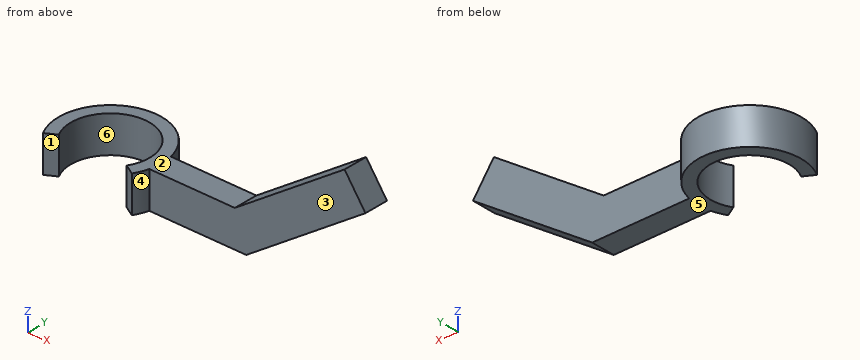
```python
from build123d import *

# Parameters (mm, degrees)
F2_DEPTH  = 15
F11_W     = 60
F11_H     = 10
F12_DEPTH = 15


with BuildPart() as f2:
    # F1 (on Top) → F2 (new body)
    with BuildSketch(Plane.XY):
        with BuildLine():
            ThreePointArc((-13.9863102711, -8.075), (0, 16.15), (13.9863102711, -8.075))
            Line((13.9863102711, -8.075), (18.31643729, -10.575))
            ThreePointArc((18.31643729, -10.575), (19.6323610311, -7.8672040995), (20.5504866122, -5))
            ThreePointArc((20.5504866122, -5), (21.15, 0), (20.5504866122, 5))
            ThreePointArc((20.5504866122, 5), (-7.8672040995, 19.6323610311), (-18.31643729, -10.575))
            Line((-18.31643729, -10.575), (-13.9863102711, -8.075))
        make_face()
        with BuildLine():
            ThreePointArc((20.5504866122, 5), (21.15, 0), (20.5504866122, -5))
            Line((20.5504866122, -5), (60.5504866122, -5))
            Line((60.5504866122, -5), (60.5504866122, 5))
            Line((60.5504866122, 5), (20.5504866122, 5))
        make_face()
    extrude(amount=F2_DEPTH)

    # F11 (on 3pt) → F12 (join)
    with BuildSketch(Plane(origin=(19.9205002513, 0, -28.4494227273), x_dir=(0.8191520443, 0, 0.5735764364), z_dir=(-0.5735764364, 0, 0.8191520443))):
        with Locations((79.6000548911, 0)):
            Rectangle(F11_W, F11_H)
    extrude(amount=F12_DEPTH)


solid = f2.part
```
Can you work these out from the model? Positions are in its coordinate system, mm. Face numbers are marked on the shaded views. A direction names the side the tool comes from. Coordinates: 2 decimals unless noted, no trailing zeros. Loops run counter-clockwise (first coordinate to the right, second up) from the corner with the lowest first, then second, coordinate; pieces in that order, holes last. Notation, with made-up numbers: (-28, 67.5) -> (30, 67.5) arc R5 cw to (30, 72.5) -> close; hole circle Ø11 at (32.25, -21.5). An arc over 180 degrees is marked (long way). Answer as a JSON object with one key per item and string values.
1) Imagine slicing it at C-C (z = 9). Please give me the cut outline in (x, y) (3 decimals).
Results:
{"outline": "(-18.316, -10.575) -> (-13.986, -8.075) arc R16.15 cw (long way) to (13.986, -8.075) -> (18.316, -10.575) arc R21.15 ccw to (20.55, -5) -> (73.404, -5) -> (73.404, 5) -> (20.55, 5) arc R21.15 ccw (long way) to start"}
2) For the marked faces 1, 2 and 3, which set-ups out of +Z, -Z, +X, -X, +Y, -Y let a thin tool reach every point of the face, with its end or its side?
Results:
{"face 1": "+Z, -Z, -Y", "face 2": "+Z, -X, +Y, -Y", "face 3": "+Z, -Z, +X, -Y"}
3) For P1, Ø14, axis at x = 54.5, z = 22, coming from the -Y side; P2, Ø12, axis at y = 15.5, z = 14, coming from the +X side; P3, Ø1, axis at y = 5, z = 16.5, coming from the +X side; P4, Ø6, axis at x = -5.5, y = 16.5, coming from the -Z side, each with a flat end and sliding along its axis, tell me the tip position at first contact or that it passes through.
Results:
{"P1": "stops at y = -5", "P2": "stops at x = 18.9", "P3": "stops at x = 84.83", "P4": "stops at z = 0"}
4) Imagine slicing it at D-D (y = 14). Please give me the cut outline in (x, z), then the cut area to 3 significant figures.
Results:
{"outline": "(-15.85, 0) -> (-8.05, 0) -> (-8.05, 15) -> (-15.85, 15) -> close; (8.05, 0) -> (15.85, 0) -> (15.85, 15) -> (8.05, 15) -> close", "area": "234 mm^2"}
5) Thinking about a two-plate mould opening in Y: for the marked faces 4, 5 and 6, which applies, pulls with the +Y half, pulls with the -Y half, needs draft (parallel to the pull), parting line crosses it, or undercut?
Results:
{"face 4": "pulls with the -Y half", "face 5": "needs draft", "face 6": "undercut"}
6) Imagine slicing it at A-A (y = 0). Please give me the cut outline in (x, z).
Results:
{"outline": "(-21.15, 0) -> (-16.15, 0) -> (-16.15, 15) -> (-21.15, 15) -> close; (16.15, 0) -> (60.55, 0) -> (109.7, 34.41) -> (101.1, 46.7) -> (55.82, 15) -> (16.15, 15) -> close"}
7) Imagine slicing it at B-B (x = 0). Please give me the cut outline in (y, z).
Results:
{"outline": "(16.15, 0) -> (21.15, 0) -> (21.15, 15) -> (16.15, 15) -> close"}
8) If I drill on line 1 (Y direction, x = 41.5, z = 10.5); line 2 (Z direction, x = 46, y = -2.5); line 3 (Y direction, x = 0, z = 8), over which ranges is the centre line in solid material (lowest first)?
Results:
{"line 1": "y = -5 to 5", "line 2": "z = 0 to 15", "line 3": "y = 16.15 to 21.15"}
